```python
from build123d import *

# Parameters (mm, degrees)
ESQUISSE1_R              = 85
BOSS_EXTRU_1_DEPTH       = 3
ESQUISSE2_W              = 32.5
ESQUISSE2_H              = 85
ENL_V_MAT_EXTRU_6_DEPTH  = 3
ESQUISSE53_R             = 2.5
ENL_V_MAT_EXTRU_21_DEPTH = 10
ESQUISSE54_R             = 2.5
ENL_V_MAT_EXTRU_22_DEPTH = 10
ESQUISSE55_R             = 6
ENL_V_MAT_EXTRU_23_DEPTH = 10


with BuildPart() as part:
    # Esquisse1 → Boss.-Extru.1 (new body)
    with BuildSketch(Plane.XY):
        with Locations((-147.95974357, 62.548931244)):
            Circle(ESQUISSE1_R)
    extrude(amount=BOSS_EXTRU_1_DEPTH)

    # Esquisse2 → Enlèv. mat.-Extru.6 (cut)
    with BuildSketch(Plane.XY):
        with BuildLine():
            Line((-199.071902892, 105.048931244), (-221.571902892, 105.048931244))
            ThreePointArc((-221.571902892, 105.048931244), (-227.739869981, 91.876928617), (-231.571902892, 77.846212492))
            Line((-231.571902892, 77.846212492), (-231.571902892, 47.251649997))
            ThreePointArc((-231.571902892, 47.251649997), (-227.739869981, 33.220933871), (-221.571902892, 20.048931244))
            Line((-221.571902892, 20.048931244), (-199.071902892, 20.048931244))
            Line((-199.071902892, 20.048931244), (-199.071902892, 105.048931244))
        make_face()
        with Locations((-80.597584249, 62.548931244)):
            Rectangle(ESQUISSE2_W, ESQUISSE2_H)
    extrude(amount=ENL_V_MAT_EXTRU_6_DEPTH, mode=Mode.SUBTRACT)


with BuildPart() as enl_v_mat_extru_6_piece_1:
    # of the separate pieces the step leaves, piece 1, a body of its own (enl_v_mat_extru_6_pieces)
    add(part.part.solids().sort_by_distance((-74.347584249, 105.048931244, 0))[0])

    # Esquisse53 → Enlèv. mat.-Extru.21 (cut)
    with BuildSketch(Plane(origin=(0, 0, 0), x_dir=(-1, 0, 0), z_dir=(0, 0, -1))):
        with Locations((190.071902892, 67.548931244)):
            Circle(ESQUISSE53_R)
        with Locations((105.847584249, 67.548931244)):
            Circle(ESQUISSE53_R)
    extrude(amount=-ENL_V_MAT_EXTRU_21_DEPTH, mode=Mode.SUBTRACT)

    # Esquisse54 → Enlèv. mat.-Extru.22 (cut)
    with BuildSketch(Plane(origin=(0, 0, 0), x_dir=(-1, 0, 0), z_dir=(0, 0, -1))):
        with Locations((195.071902892, 117.048931244)):
            Circle(ESQUISSE54_R)
        with Locations(Location((100.847584249, 117.048931244, 0), (0, 0, 180))):
            Circle(ESQUISSE54_R)
    extrude(amount=-ENL_V_MAT_EXTRU_22_DEPTH, mode=Mode.SUBTRACT)

    # Esquisse55 → Enlèv. mat.-Extru.23 (cut)
    with BuildSketch(Plane(origin=(0, 0, 0), x_dir=(-1, 0, 0), z_dir=(0, 0, -1))):
        with Locations((147.95974357, 62.548931244)):
            Circle(ESQUISSE55_R)
    extrude(amount=-ENL_V_MAT_EXTRU_23_DEPTH, mode=Mode.SUBTRACT)


with BuildPart() as enl_v_mat_extru_6_piece_2:
    # of the separate pieces the step leaves, piece 2, a body of its own (enl_v_mat_extru_6_pieces)
    add(part.part.solids().sort_by_distance((-64.347584249, 47.251649997, 0))[0])


with BuildPart() as enl_v_mat_extru_6_piece_3:
    # of the separate pieces the step leaves, piece 3, a body of its own (enl_v_mat_extru_6_pieces)
    add(part.part.solids().sort_by_distance((-231.571902892, 77.846212492, 0))[0])


solid = enl_v_mat_extru_6_piece_1.part
```
Input: part model. Units: mm. Frame: model coordinates. Round coordinates to 2 decimals unless told otherwise and drop trailing zeros. Write each loop counter-clockwise with the first axis right and the second up, starting at its lowest first coordinate (ties: lowest second). Pieces come first, ordered by that corner, then holes. Notation, with made-up numbers: M 32,50 L 81,50 A20 ccw 81,88 Z; hole C 63.5,-4 d8. An arc over 180 degrees is marked long. Write each question's results on one line, items separated by ' | '.
Q1. Section query D-D (x = -93). Return loops of the section in (y, z), and give its area (3 significant figures).
Results:
outline: M -2.29,0 L 20.05,0 L 20.05,3 L -2.29,3 Z; M 105.05,0 L 127.39,0 L 127.39,3 L 105.05,3 Z | area: 134 mm^2
Q2. Section query A-A (x = -148). Return loops of the section in (y, z).
Results:
outline: M -22.45,0 L 56.55,0 L 56.55,3 L -22.45,3 Z; M 68.55,0 L 147.55,0 L 147.55,3 L 68.55,3 Z
Q3. Section query B-B (z = 0.5). Return loops of the section in (x, y), and give its area (3 significant figures).
Results:
outline: M -221.57,20.05 A85 ccw -74.35,20.05 L -96.85,20.05 L -96.85,105.05 L -74.35,105.05 A85 ccw -221.57,105.05 L -199.07,105.05 L -199.07,20.05 Z; hole C -195.07,117.05 d5; hole C -190.07,67.55 d5; hole C -147.96,62.55 d12; hole C -105.85,67.55 d5; hole C -100.85,117.05 d5 | area: 17,400 mm^2
Q4. Line query: line 1 along X through (y, z) = (66.5, 0.95); line 2 along Y through (x, z) = (-193.5, 2.3); line 3 along X through (y, z) = (76.5, 2.55). Output: solid intervals per line, ascending.
Results:
line 1: x = -199.07 to -192.34, -187.8 to -152.48, -143.44 to -108.12, -103.58 to -96.85 | line 2: y = -9.22 to 115.1, 118.99 to 134.32 | line 3: x = -199.07 to -96.85
Q5. Draft query along Y for faces 1 (the face through (-146.71, 147.54, 1.48)), 2 (the face through (-149.21, -22.44, 1.48)), 3 (the face through (-133, 64, 0)), 4 (the face through (-143.198, 58.898, 1.479)). Return one class per face: released by +Y, released by -Y, zero draft, split by the parting line, or undercut.
Results:
face 1: released by +Y | face 2: released by -Y | face 3: zero draft | face 4: undercut
Q6. Pin query (flat end, axial travel): P1, Ø0.9, axis at x = -90.5, z = 1.5, coming from the +Y side; P2, Ø4, axis at x = -190.07, y = 67.55, coming from the -Z side; P3, Ø1.5, axis at x = -211, z = 1, coming from the -Y side; P4, Ø0.9, axis at x = -206.5, z = 1, coming from the +Y side. Return the tip coordinate at first contact, or that it passes through.
Results:
P1: stops at y = 125.6 | P2: passes through | P3: stops at y = 4.71 | P4: stops at y = 124.6
Q7. Section query C-C (y = 80). Return loops of the section in (x, z).
Results:
outline: M -199.07,0 L -96.85,0 L -96.85,3 L -199.07,3 Z
